Check sheet for the drawn part. Datum: minimum x, y, z corner. Units: mm. A direction names the side the tool comes from. Round coordinates to 2 decimals unless told otherwise and drop trailing zeros. Order: outer loops, then holes, each group sorted by start corner. A loop starts at its lowest first (then second) coordinate and runs counter-clockwise, first axis right, second up. Notation, with made-up numbers: (31, 69.5) -> (84, 69.5) arc R31 cw to (84, 99.5) -> close; hole circle Ø7 at (-25.5, 13). An arc over 180 degrees is marked (long way). Answer as CSV lines item,"result". Start each with the question number.
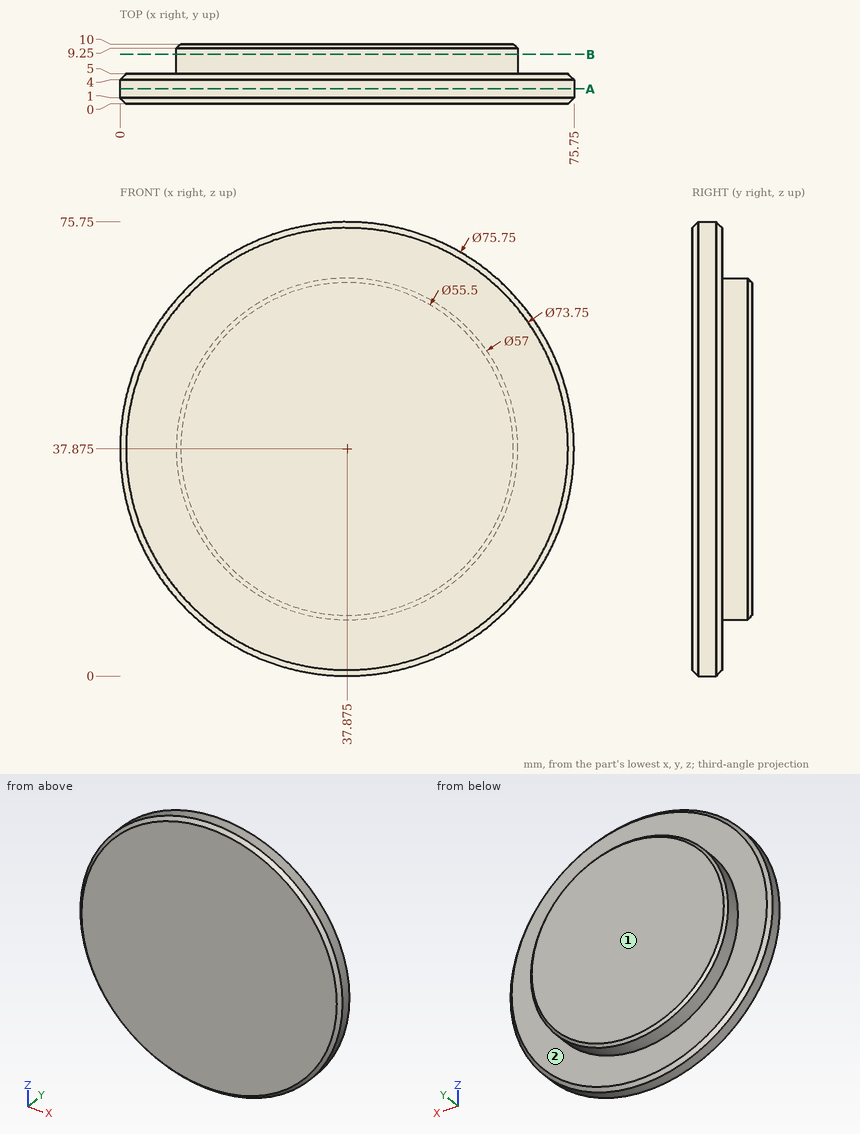
1) Section check B-B on y = 8.25. Record the cut outline in (x, z) (3 decimals), then the cut area to 3 significant figures.
2) Material ranges on line 1 along X through (y, z) = (2.25, 39); line 2 along Y through (x, z) = (16, 65); line 3 along Z through (x, y) = (38.5, 7.75), recorded low to high.
3) Section check A-A on y = 2.5. Record the cut outline in (x, z) (3 decimals), then the cut area to 3 significant figures.
4) Depth check by flat-ended pin: pin 1 Ø3 at (x, y) = (44, 8) entering from +Z; pin 2 Ø3 at (y, z) = (2.5, 59) entering from +X; pin 3 Ø4 at (y, z) = (2.5, 52) entering from -X. Enter the tip coordinate at first touch or a pass-through.
5) Access from +Z, -Z, +X, -X, +Y, -Y to the whole of each face (thin tool, end or side, straight path). Record for the marked faces 1 and 2.
Solutions:
1,outline,"circle Ø57 at (37.875, 37.875)"
1,area,"2,550 mm^2"
2,line 1,"x = 0.02 to 75.73"
2,line 2,"y = 0 to 5"
2,line 3,"z = 9.38 to 66.37"
3,outline,"circle Ø75.75 at (37.875, 37.875)"
3,area,"4,510 mm^2"
4,pin 1,"stops at z = 66"
4,pin 2,"stops at x = 70.27"
4,pin 3,"stops at x = 1.99"
5,face 1,"+Z, -Z, +X, -X, +Y"
5,face 2,"+Y"
